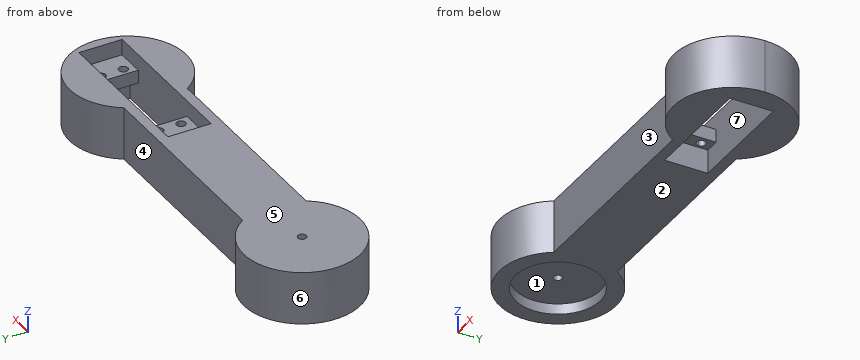
```python
from build123d import *

# Parameters (mm, degrees)
BOSS_EXTRUDE1_DEPTH = 25
SKETCH19_R          = 20
CUT_EXTRUDE14_DEPTH = 5
SKETCH22_R          = 2
CUT_EXTRUDE17_DEPTH = 20
SKETCH23_W          = 54.5
SKETCH23_H          = 20.4
SKETCH23_W_2        = 40.6
CUT_EXTRUDE18_DEPTH = 11.3
CUT_EXTRUDE19_DEPTH = 13.7
SKETCH25_W          = 7.5
SKETCH25_H          = 20.4
CUT_EXTRUDE20_DEPTH = 13.5
CUT_EXTRUDE21_DEPTH = 20
SKETCH27_R          = 2.15
CUT_EXTRUDE22_DEPTH = 12


with BuildPart() as part:
    # Sketch1 → Boss-Extrude1 (new body)
    with BuildSketch(Plane.XY):
        with BuildLine():
            ThreePointArc((172.5, 0), (152.823244805, 26.363741023), (121.951138857, 15))
            Line((121.951138857, 15), (145, 15))
            Line((145, 15), (145, -15))
            Line((145, -15), (121.951138857, -15))
            ThreePointArc((121.951138857, -15), (152.823244805, -26.363741023), (172.5, 0))
        make_face()
        with BuildLine():
            Line((145, 15), (121.951138857, 15))
            ThreePointArc((121.951138857, 15), (117.5, 0), (121.951138857, -15))
            Line((121.951138857, -15), (145, -15))
            Line((145, -15), (145, 15))
        make_face()
        with BuildLine():
            Line((121.951138857, 15), (23.048861143, 15))
            ThreePointArc((23.048861143, 15), (26.363741023, 7.823244805), (27.5, 0))
            ThreePointArc((27.5, 0), (26.363741023, -7.823244805), (23.048861143, -15))
            Line((23.048861143, -15), (121.951138857, -15))
            ThreePointArc((121.951138857, -15), (117.5, 0), (121.951138857, 15))
        make_face()
        with BuildLine():
            ThreePointArc((13.228756555, -15), (-20, 0), (13.228756555, 15))
            Line((13.228756555, 15), (23.048861143, 15))
            ThreePointArc((23.048861143, 15), (-27.5, 0), (23.048861143, -15))
            Line((23.048861143, -15), (13.228756555, -15))
        make_face()
        with BuildLine():
            Line((23.048861143, 15), (13.228756555, 15))
            ThreePointArc((13.228756555, 15), (18.228756555, 8.228756555), (20, 0))
            ThreePointArc((20, 0), (18.228756555, -8.228756555), (13.228756555, -15))
            Line((13.228756555, -15), (23.048861143, -15))
            ThreePointArc((23.048861143, -15), (26.363741023, -7.823244805), (27.5, 0))
            ThreePointArc((27.5, 0), (26.363741023, 7.823244805), (23.048861143, 15))
        make_face()
        with BuildLine():
            Line((0, -15), (0, 15))
            Line((0, 15), (13.228756555, 15))
            ThreePointArc((13.228756555, 15), (-20, 0), (13.228756555, -15))
            Line((13.228756555, -15), (0, -15))
        make_face()
        with BuildLine():
            Line((13.228756555, 15), (0, 15))
            Line((0, 15), (0, -15))
            Line((0, -15), (13.228756555, -15))
            ThreePointArc((13.228756555, -15), (18.228756555, -8.228756555), (20, 0))
            ThreePointArc((20, 0), (18.228756555, 8.228756555), (13.228756555, 15))
        make_face()
    extrude(amount=BOSS_EXTRUDE1_DEPTH)

    # Sketch19 → Cut-Extrude14 (cut)
    with BuildSketch(Plane(origin=(0, 0, 0), x_dir=(-1, 0, 0), z_dir=(0, 0, -1))):
        Circle(SKETCH19_R)
    extrude(amount=-CUT_EXTRUDE14_DEPTH, mode=Mode.SUBTRACT)

    # Sketch22 → Cut-Extrude17 (cut)
    with BuildSketch(Plane.XY.offset(25)):
        Circle(SKETCH22_R)
    extrude(amount=-CUT_EXTRUDE17_DEPTH, mode=Mode.SUBTRACT)

    # Sketch23 → Cut-Extrude18 (cut)
    with BuildSketch(Plane(origin=(0, 0, 0), x_dir=(-1, 0, 0), z_dir=(0, 0, -1))):
        with Locations((-134, 0)):
            Rectangle(SKETCH23_W, SKETCH23_H)
        with Locations((-134, 0)):
            Rectangle(SKETCH23_W_2, SKETCH23_H)
    extrude(amount=-CUT_EXTRUDE18_DEPTH, mode=Mode.SUBTRACT)

    # Sketch24 → Cut-Extrude19 (cut)
    with BuildSketch(Plane(origin=(0, 0, 11.3), x_dir=(-1, 0, 0), z_dir=(0, 0, -1))):
        Polygon((-154.3, -0.627488927), (-154.3, -10.2), (-113.7, -10.2), (-113.7, 10.2), (-154.3, 10.2), align=None)
    extrude(amount=-CUT_EXTRUDE19_DEPTH, mode=Mode.SUBTRACT)

    # Sketch25 → Cut-Extrude20 (cut)
    with BuildSketch(Plane.ZY.offset(-154.3)):
        with Locations((21.25, 0)):
            Rectangle(SKETCH25_W, SKETCH25_H)
    extrude(amount=-CUT_EXTRUDE20_DEPTH, mode=Mode.SUBTRACT)

    # Sketch26 → Cut-Extrude21 (cut)
    with BuildSketch(Plane(origin=(113.7, 0, 0), x_dir=(0, 0, -1), z_dir=(1, 0, 0))):
        Polygon((-25, 10.2), (-25, -10.2), (-17.5, -10.2), (-17.5, 10.2), (-21.25, 10.2), align=None)
    extrude(amount=-CUT_EXTRUDE21_DEPTH, mode=Mode.SUBTRACT)

    # Sketch27 → Cut-Extrude22 (cut)
    with BuildSketch(Plane(origin=(0, 0, 11.3), x_dir=(-1, 0, 0), z_dir=(0, 0, -1))):
        with BuildLine():
            ThreePointArc((-107.85, 5.25), (-110, 7.4), (-112.15, 5.25))
            Line((-112.15, 5.25), (-110, 5.25))
            Line((-110, 5.25), (-110, 3.1))
            ThreePointArc((-110, 3.1), (-108.47972042, 3.72972042), (-107.85, 5.25))
        make_face()
        with BuildLine():
            Line((-110, 5.25), (-112.15, 5.25))
            ThreePointArc((-112.15, 5.25), (-111.52027958, 3.72972042), (-110, 3.1))
            Line((-110, 3.1), (-110, 5.25))
        make_face()
        with BuildLine():
            ThreePointArc((-110, -3.1), (-111.52027958, -3.72972042), (-112.15, -5.25))
            Line((-112.15, -5.25), (-110, -5.25))
            Line((-110, -5.25), (-110, -3.1))
        make_face()
        with BuildLine():
            Line((-110, -5.25), (-112.15, -5.25))
            ThreePointArc((-112.15, -5.25), (-110, -7.4), (-107.85, -5.25))
            ThreePointArc((-107.85, -5.25), (-108.47972042, -3.72972042), (-110, -3.1))
            Line((-110, -3.1), (-110, -5.25))
        make_face()
        with BuildLine():
            ThreePointArc((-155.85, 5.25), (-159.52027958, 6.77027958), (-158, 3.1))
            Line((-158, 3.1), (-158, 5.25))
            Line((-158, 5.25), (-155.85, 5.25))
        make_face()
        with BuildLine():
            Line((-158, 5.25), (-158, 3.1))
            ThreePointArc((-158, 3.1), (-156.47972042, 3.72972042), (-155.85, 5.25))
            Line((-155.85, 5.25), (-158, 5.25))
        make_face()
        with Locations((-158, -5.25)):
            Circle(SKETCH27_R)
    extrude(amount=-CUT_EXTRUDE22_DEPTH, mode=Mode.SUBTRACT)


solid = part.part
```
Geometry check sheet. Reference: the model listing, model coordinates, mm. Face numbers are marked on the shaded views. A direction names the side the tool comes from. Coordinates: 2 decimals unless noted, no trailing zeros. Loops run counter-clockwise (first coordinate to the right, second up) from the corner with the lowest first, then second, coordinate; pieces in that order, holes last. Notation, with made-up numbers: (33.25, 13.5) - (90.25, 13.5) arc R16 cw to (90.25, 18.5) - close; hole circle Ø7 at (84.5, 43.25). An arc over 180 degrees is marked (long way). One line per item, written item: value. Start each with the question number.
(1) Tool access check on the marked faces 1, 2, 3 and 4. Record the directions out of +Z, -Z, +X, -X, +Y, -Y that give a thin tool (end or side, any length) a straight path to the whole face; none if there is none.
(2) Cross-section at A-A on x = 0. Enter the section's corners in (y, z).
(3) Material ranges on line 1 (Y direction, x = 158, z = 15); line 2 (X direction, y = -16.5, z = 4); line 3 (X direction, y = 5.25, z = 15), recorded low to high. Write a range as [from, to].
(4) Cross-section at C-C on x = 100.5. Enter the section's corners in (y, z).
(5) Mould release check, pull along X, two halves, no side actions. Record for the marked faces 5, 6 and 7: released by +X, released by -X, zero draft, split by the parting line, or undercut.
(6) Cross-section at D-D on z = 21.75. Enter the section's corners in (x, y).
(7) Depth check by flat-ended pin: P1, Ø3.5, axis at x = 0, y = 0, coming from the +Z side; P2, Ø1, axis at y = -20, z = 8.5, coming from the +X side; P3, Ø3.5, axis at y = 5, z = 8, coming from the +X side; P4, Ø11, axis at x = 159.5, y = 4.5, coming from the +Z side. Enter the tip coordinate at first touch or a pass-through.
(8) Cross-section at B-B on z = 13.5. Enter the section's corners in (x, y), plus the area to 3 significant figures.
Results below:
1. face 1: -Z
1. face 2: -Z, +X, -X, +Y, -Y
1. face 3: +Z, -Z, -Y
1. face 4: +Z, -Z, +Y
2. outline: (-27.5, 0) - (-20, 0) - (-20, 5) - (-2, 5) - (-2, 25) - (-27.5, 25) - close; (2, 5) - (20, 5) - (20, 0) - (27.5, 0) - (27.5, 25) - (2, 25) - close
3. line 1: y = [-24.23, -7.4], [-3.1, 3.1], [7.4, 24.23]
3. line 2: x = [-22, -11.3], [11.3, 22], [123, 167]
3. line 3: x = [-26.99, 107.85], [112.15, 113.7], [154.3, 155.85], [160.15, 171.99]
4. outline: (-15, 0) - (15, 0) - (15, 25) - (10.2, 25) - (10.2, 17.5) - (-10.2, 17.5) - (-10.2, 25) - (-15, 25) - close
5. face 5: zero draft
5. face 6: undercut
5. face 7: undercut
6. outline: (23.05, -15) - (121.95, -15) arc R27.5 ccw (long way) to (121.95, 15) - (23.05, 15) arc R27.5 ccw (long way) to start; hole circle Ø4 at (0, 0); hole (93.7, -10.2) - (167.8, -10.2) - (167.8, 10.2) - (93.7, 10.2) - close
7. P1: passes through
7. P2: stops at x = 164.39
7. P3: stops at x = 172.31
7. P4: stops at z = 17.5
8. outline: (23.05, -15) - (121.95, -15) arc R27.5 ccw (long way) to (121.95, 15) - (23.05, 15) arc R27.5 ccw (long way) to start; hole circle Ø4 at (0, 0); hole circle Ø4.3 at (110, -5.25); hole circle Ø4.3 at (110, 5.25); hole (113.7, -10.2) - (154.3, -10.2) - (154.3, 10.2) - (113.7, 10.2) - close; hole circle Ø4.3 at (158, -5.25); hole circle Ø4.3 at (158, 5.25)
8. area: 6,640 mm2
